Check sheet for the drawn part. Datum: minimum x, y, z corner. Units: mm. Coordinates: 2 decimals unless noted, no trailing zeros. Write each loop counter-clockwise with the first axis right and the second up, starting at its lowest first coordinate (ties: lowest second). Pieces come first, ordered by that corner, then holes. Notation, with made-up numbers: (-25, 72.5) -> (-8, 72.5) arc R32 ccw to (-8, 102.5) -> close; hole circle Ø8 at (80.5, 67). An arc over 180 degrees is marked (long way). Answer in a Markdown table with one row per item.
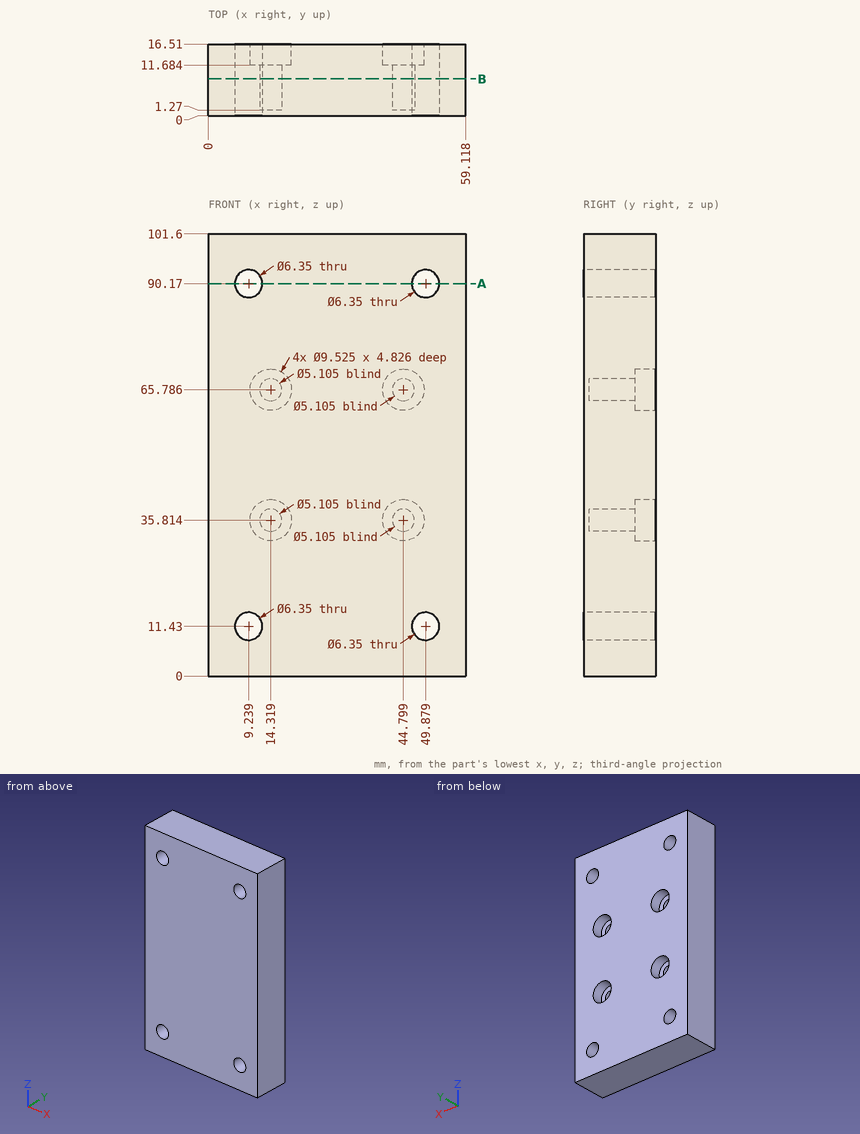
1. Material ranges on probe 1 along Z at (x, y) = (9, 6.5) (1 decimal); probe 2 along X at (y, z) = (10.5, 90.17) (1 decimal); probe 3 along Z at (x, y) = (43, 4) (1 decimal), recorded low to high. Write a range as from..to.
Findings below:
| item | result |
|---|---|
| probe 1 | z = 0..8.3, 14.6..87, 93.3..101.6 |
| probe 2 | x = 0..6.1, 12.4..46.7, 53.1..59.1 |
| probe 3 | z = 0..34, 37.6..64, 67.6..101.6 |
2. Go/stop test with flat-tipped pins: pin 1 (3 mm diameter, centred on x = 45.5, z = 38, fed in from +Y); pin 2 (4.5 mm diameter, centred on x = 14.32, z = 65.79, fed in from +Y). Record where each tip stops, or that it passes through.
Findings below:
| item | result |
|---|---|
| pin 1 | stops at y = 11.68 |
| pin 2 | stops at y = 1.27 |
3. Sectioned sample at A-A, the plane z = 90.17. Record the cut outline in (x, y) (1 decimal).
Findings below:
| item | result |
|---|---|
| outline | (0, 0) -> (6.1, 0) -> (6.1, 16.5) -> (0, 16.5) -> close; (12.4, 0) -> (46.7, 0) -> (46.7, 16.5) -> (12.4, 16.5) -> close; (53.1, 0) -> (59.1, 0) -> (59.1, 16.5) -> (53.1, 16.5) -> close |
4. Sectioned sample at B-B, the plane y = 8.5. Count the separate pieces of the cut face and the enclosed holes in it, and give its area (3 significant figures).
Findings below:
| item | result |
|---|---|
| separate pieces | 1 |
| enclosed holes | 8 |
| area | 5,800 mm² |
